from build123d import *

# Parameters (mm, degrees)
SKETCH1_W           = 40
SKETCH1_H           = 275
BOSS_EXTRUDE1_DEPTH = 3
SKETCH2_R           = 1.7
CUT_EXTRUDE1_DEPTH  = 139.979315008
FILLET1_R           = 20
CUT_EXTRUDE2_DEPTH  = 139.979315008


with BuildPart() as part:
    # Sketch1 → Boss-Extrude1 (new body)
    with BuildSketch(Plane(origin=(0, 0, 0), x_dir=(1, 0, 0), z_dir=(0, 1, 0))):
        Rectangle(SKETCH1_W, SKETCH1_H)
    extrude(amount=BOSS_EXTRUDE1_DEPTH)

    # Sketch2 → Cut-Extrude1 (cut, through all)
    with BuildSketch(Plane(origin=(0, 3, 0), x_dir=(1, 0, 0), z_dir=(0, 1, 0))):
        with Locations(Location((-11, 128.5, 0), (0, 0, 270))):
            Circle(SKETCH2_R)
        with Locations(Location((-11, 106.5, 0), (0, 0, 270))):
            Circle(SKETCH2_R)
        with Locations(Location((11, 128.5, 0), (0, 0, 270))):
            Circle(SKETCH2_R)
        with Locations(Location((11, 106.5, 0), (0, 0, 270))):
            Circle(SKETCH2_R)
    extrude(amount=-CUT_EXTRUDE1_DEPTH, mode=Mode.SUBTRACT)

    # Fillet1
    fillet1_edges = [part.edges().sort_by_distance(p)[0] for p in [
        (-20, 1.5, 137.5),
        (20, 1.5, 137.5),
    ]]
    fillet(fillet1_edges, radius=FILLET1_R - 0.0001)  # a hair under: the kernel refuses the full size

    # Sketch3 → Cut-Extrude2 (cut, through all)
    with BuildSketch(Plane(origin=(0, 3, 0), x_dir=(1, 0, 0), z_dir=(0, 1, 0))):
        with BuildLine():
            Line((-3, 22.5), (-3, -117.5))
            ThreePointArc((-3, -117.5), (0, -120.5), (3, -117.5))
            Line((3, -117.5), (3, 22.5))
            ThreePointArc((3, 22.5), (0, 25.5), (-3, 22.5))
        make_face()
    extrude(amount=-CUT_EXTRUDE2_DEPTH, mode=Mode.SUBTRACT)


solid = part.part
Design review of the part built by this model. Coordinates are the model's own, in mm. Round coordinates to 2 decimals unless told otherwise and drop trailing zeros. Loops run counter-clockwise (first coordinate to the right, second up) from the corner with the lowest first, then second, coordinate; pieces in that order, holes last. Notation, with made-up numbers: (57.5, 78.5) - (64.5, 78.5) arc R22 cw to (64.5, 86.5) - close; hole circle Ø11 at (59.25, 52). An arc over 180 degrees is marked (long way). One line per item, written item: value. Start each with the question number.
1) Consider section B-B on z = 46. Give the boundary of the cut face in (x, y).
2) Consider section C-C on x = -16. Give the boundary of the cut face in (y, z), then the cut area to 3 significant figures.
3) Consider section A-A on y = 1.65. Give the number of separate pieces and of enclosed holes in the cut face, then the cut area to 3 significant figures.
4) Insertion check: pin 1 Ø2.5 at (x, z) = (11, -128.5) entering from -Y; pin 2 Ø12 at (x, z) = (-0.5, 89.5) entering from -Y. Each pin has a flat end and moves straight along its axis. Give the tip position at first contact, or say it passes through.
5) To check wall thickness, follow L1, parallel to X at y = 2, z = -106.5; L2, parallel to X at y = 1.15, z = 110.5; L3, parallel to X at y = 1.15, z = -108. State the ranges of each line that lie inside material, in increasing order. Write a range as from..to.
Reported:
1. outline: (-20, 0) - (-3, 0) - (-3, 3) - (-20, 3) - close; (3, 0) - (20, 0) - (20, 3) - (3, 3) - close
2. outline: (0, -137.5) - (3, -137.5) - (3, 129.5) - (0, 129.5) - close
2. area: 801 mm^2
3. separate pieces: 1
3. enclosed holes: 5
3. area: 9,920 mm^2
4. pin 1: passes through
4. pin 2: stops at y = 0
5. L1: x = -20..-12.7, -9.3..9.3, 12.7..20
5. L2: x = -20..-3, 3..20
5. L3: x = -20..-11.8, -10.2..10.2, 11.8..20
